Check sheet for the drawn part. Datum: minimum x, y, z corner. Units: mm. Round coordinates to 2 decimals unless told otherwise and drop trailing zeros. Write each loop counter-clockwise with the first axis right and the second up, starting at its lowest first coordinate (ties: lowest second). Pieces come first, ordered by that corner, then holes. Notation, with made-up numbers: (83, -17.75) - (125, -17.75) arc R13 cw to (125, 1.25) - close; hole circle Ø3 at (78, 86.25). An arc over 180 degrees is marked (long way). Answer as a JSON object with one key per item and string values. Group by question number.
1) Go/stop test with flat-tipped pins: pin 1 Ø0.5 at (x, y) = (9, 6.5) entering from +Z; pin 2 Ø0.8 at (x, y) = (9, 7.5) entering from -Z; pin 3 Ø3 at (y, z) = (7, 12) entering from +X; pin 4 Ø6 at (x, y) = (6, 12) entering from -Z. Record where each tip stops, or that it passes through.
2) Thickness scan on line 1 (Y direction, x = 7, z = 5.25); line 2 (X direction, y = 7, z = 15.75); line 3 (Z direction, x = 10, y = 13). Record the ranges inside material, lowest first.
3) Section check A-A (x = 7). Enter the section's corners in (y, z), then the cut area to 3 significant figures.
4) Section check B-B (y = 7). Enter the section's corners in (x, z), then the cut area to 3 significant figures.
5) Section check D-D (x = 10). Enter the section's corners in (y, z).
6) Mould release check, pull along Y, two halves, no side actions. Record for the marked faces 1, 2 and 3: +Y half, -Y half, draft (parallel to the pull), parting line (faces both ways), or undercut.
7) Section check C-C (z = 2). Enter the section's corners in (x, y).
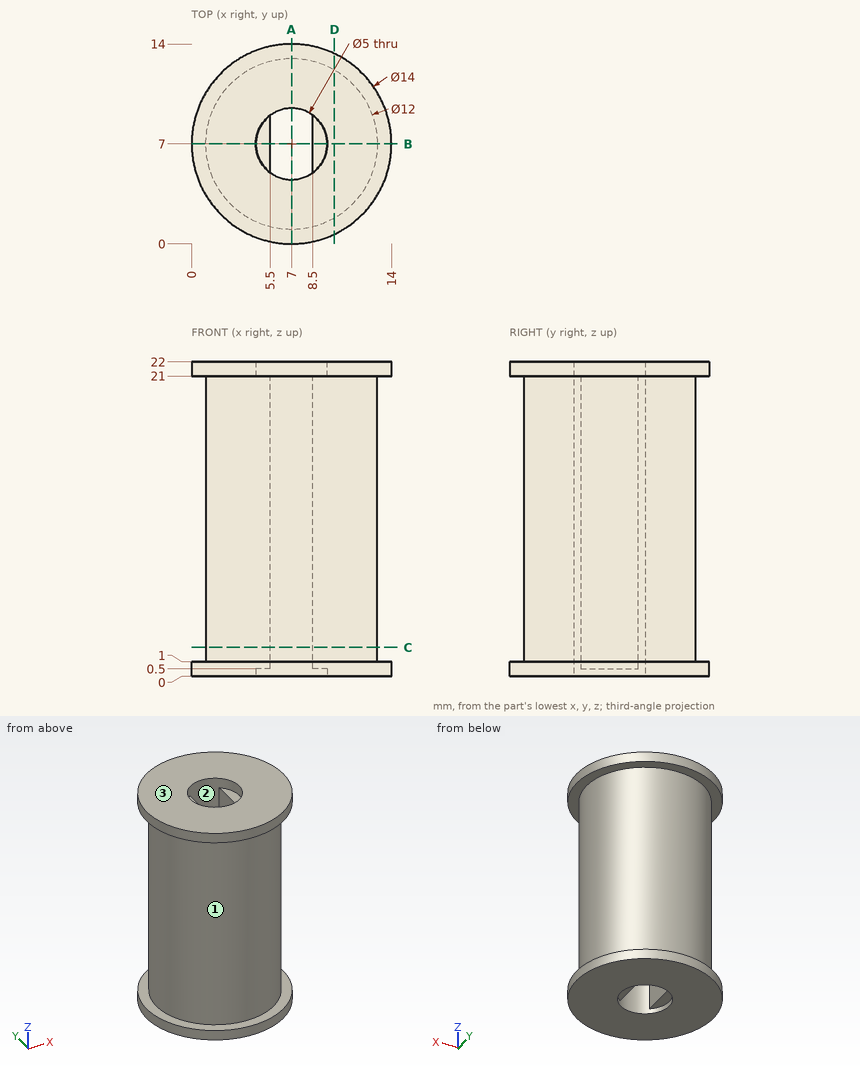
Returned:
{
 "1": {"pin 1": "z = 21", "pin 2": "z = 0.5", "pin 3": "x = 13", "pin 4": "z = 0"},
 "2": {"line 1": "1 to 4.5, 9.5 to 13", "line 2": "1 to 5.5, 8.5 to 13", "line 3": "0 to 1, 21 to 22"},
 "3": {"outline": "(0, 0) - (4.5, 0) - (4.5, 22) - (0, 22) - (0, 21) - (1, 21) - (1, 1) - (0, 1) - close; (9.5, 0) - (14, 0) - (14, 1) - (13, 1) - (13, 21) - (14, 21) - (14, 22) - (9.5, 22) - close", "area": "158 mm2"},
 "4": {"outline": "(0, 0) - (4.5, 0) - (4.5, 0.5) - (5.5, 0.5) - (5.5, 21) - (4.5, 21) - (4.5, 22) - (0, 22) - (0, 21) - (1, 21) - (1, 1) - (0, 1) - close; (8.5, 0.5) - (9.5, 0.5) - (9.5, 0) - (14, 0) - (14, 1) - (13, 1) - (13, 21) - (14, 21) - (14, 22) - (9.5, 22) - (9.5, 21) - (8.5, 21) - close", "area": "199 mm2"},
 "5": {"outline": "(0.68, 0) - (13.32, 0) - (13.32, 1) - (12.2, 1) - (12.2, 21) - (13.32, 21) - (13.32, 22) - (0.68, 22) - (0.68, 21) - (1.8, 21) - (1.8, 1) - (0.68, 1) - close"},
 "6": {"face 1": "parting line", "face 2": "undercut", "face 3": "draft"},
 "7": {"outline": "circle Ø12 at (7, 7); hole (5.5, 5) arc R2.5 ccw to (8.5, 5) - (8.5, 9) arc R2.5 ccw to (5.5, 9) - close"}
}
